Here's the drawing with two shaded views (mm, measured from the low corner). I have some questions. A direction names the side the tool comes from. Give positions to 0.01 mm unless a question says otherwise; leave off trailing zeros. Loops run counter-clockwise (first coordinate to the right, second up) from the corner with the lowest first, then second, coordinate; pieces in that order, holes last.
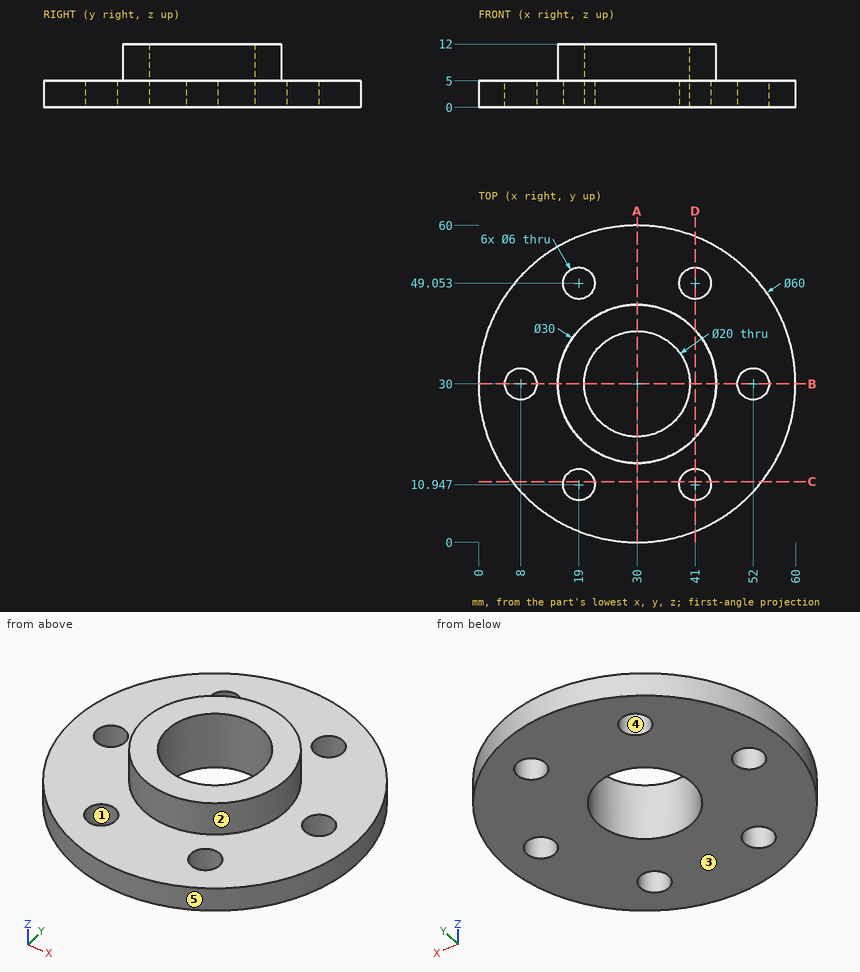
(1) Suppose I cut it at C-C on y = 11.5. List the corners of the cut face in (x, z) for me.
Returned:
outline: (6.38, 0) - (16.05, 0) - (16.05, 5) - (6.38, 5) - close; (21.95, 0) - (38.05, 0) - (38.05, 5) - (21.95, 5) - close; (43.95, 0) - (53.62, 0) - (53.62, 5) - (43.95, 5) - close
(2) Suppose I cut it at B-B on y = 30. List the corners of the cut face in (x, z) for me.
Returned:
outline: (0, 0) - (5, 0) - (5, 5) - (0, 5) - close; (11, 0) - (20, 0) - (20, 12) - (15, 12) - (15, 5) - (11, 5) - close; (40, 0) - (49, 0) - (49, 5) - (45, 5) - (45, 12) - (40, 12) - close; (55, 0) - (60, 0) - (60, 5) - (55, 5) - close
(3) Please list where these lines run through material, in increasing order: probe 1 along Y at (x, z) = (41, 3.7); probe 2 along Y at (x, z) = (30, 4.5); probe 3 along Z at (x, y) = (45, 9.5).
Returned:
probe 1: y = 2.09 to 7.95, 13.95 to 46.05, 52.05 to 57.91
probe 2: y = 0 to 20, 40 to 60
probe 3: z = 0 to 5
(4) Suppose I cut it at D-D on x = 41. List the corners of the cut face in (y, z) for me.
Returned:
outline: (2.09, 0) - (7.95, 0) - (7.95, 5) - (2.09, 5) - close; (13.95, 0) - (46.05, 0) - (46.05, 5) - (40.2, 5) - (40.2, 12) - (19.8, 12) - (19.8, 5) - (13.95, 5) - close; (52.05, 0) - (57.91, 0) - (57.91, 5) - (52.05, 5) - close
(5) Suppose I cut it at A-A on x = 30. List the corners of the cut face in (y, z) for me, plus the area to 3 significant figures.
Returned:
outline: (0, 0) - (20, 0) - (20, 12) - (15, 12) - (15, 5) - (0, 5) - close; (40, 0) - (60, 0) - (60, 5) - (45, 5) - (45, 12) - (40, 12) - close
area: 270 mm2
(6) Thinking about a two-plate mould opening in X: for the marked faces 3, 4 and 5, which applies, pulls with the +X half, pulls with the -X half, needs draft (parallel to the pull), parting line crosses it, or undercut?
Returned:
face 3: needs draft
face 4: undercut
face 5: parting line crosses it
(7) Which directions (+Z, -Z, +X, -X, +Y, -Y) give clear straight access to the entire face, cutting with the end or side of a thin tool? Please do the marked faces 1 and 2.
Returned:
face 1: +Z, -Z
face 2: +Z
(8) Will these pins go through, and if not, where does the flat tip stop? P1, Ø1, axis at x = 48.5, y = 53.5, coming from the +Z side; P2, Ø2, axis at y = 43.5, z = 10, coming from the -X side; P3, Ø4, axis at y = 38, z = 1.5, coming from the +X side.
Returned:
P1: stops at z = 5
P2: stops at x = 21.71
P3: stops at x = 59.39
